Can you work these out from the model? Positions are in its coordinate system, mm. Face numbers are marked on the shaded views. A direction names the side the tool comes from. Give positions to 0.01 mm unless a question says otherwise; leave off trailing zeros. Order: outer loops, then holes, each group sorted by start corner. A loop starts at its lowest first (then second) coordinate and runs counter-clockwise, first axis right, second up. Notation, with made-up numbers: M 13.5,-23 L 55.5,-23 A24 ccw 55.5,1 Z; hole C 36.25,1 d7. An arc over 180 degrees is marked long. One line per question, with ' | ' between items. Start each with the question number.
1) Please list where these lines run through material, in increasing order: line 1 along Y through (x, z) = (0, 8.5); line 2 along X through (y, z) = (-6, 30) (3 decimals); line 3 along Y through (x, z) = (28, 38) (3 decimals). Write a range as [from, to].
2) If we section it at A-A, the plane x = 45: Please give me the cut outline in (y, z) (3 decimals).
3) Thinking about a two-plate mould opening in Y: for the marked faces 1, 2 and 3, which applies, +Y half, -Y half, draft (parallel to the pull), parting line (faces both ways), or undercut?
4) I'm going to push flat-ended pins straight in: pin 1 Ø5 at (y, z) = (5.5, 8) entering from -X; pin 2 Ø1.5 at (x, y) = (-3.5, -18) entering from +Z; pin 3 Ø15 at (y, z) = (0.5, 28.5) entering from +X (3 decimals); pin 4 Ø5 at (x, z) = (-16.5, 39.5) entering from -Y (1 decimal). Where does each tip first touch, or does it pass through?
5) If we section it at C-C, the plane z = 41: Please give me the cut outline in (x, y) (3 decimals).
6) For the marked faces 4, 5, 6, 7 and 8, which set-ups out of +Z, -Z, +X, -X, +Y, -Y let a thin tool reach every point of the face, with its end or its side?
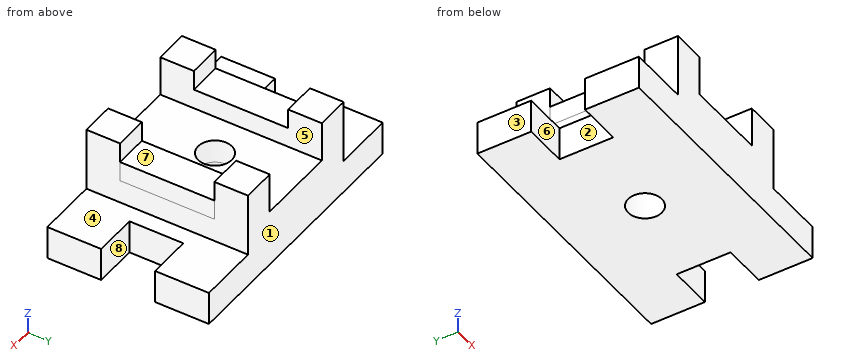
```python
from build123d import *

# Parameters (mm, degrees)
F1_DEPTH = 15.875
F2_W     = 69.85
F2_H     = 76.2
F2_R     = 7.9375
F3_DEPTH = 11.1125
F4_DEPTH = 15.876
F5_W     = 15.875
F5_H     = 15.875
F6_DEPTH = 19.05
F7_W     = 15.875
F7_H     = 44.45
F8_DEPTH = 9.525


# Not quite as in the source:
# - a length typed as a fraction of an inch, garbled in the dataset ("3 / 203.2 mm" for 3/8 in), is restored


with BuildPart() as f1:
    # F0 (on Top) → F1 (new body)
    with BuildSketch(Plane.XY):
        Polygon((63.5, 12.7), (63.5, 38.1), (-63.5, 38.1), (-63.5, 12.7), (-42.8498, 12.7), (-42.8498, -12.7), (-63.5, -12.7), (-63.5, -38.1), (63.5, -38.1), (63.5, -12.7), (42.8498, -12.7), (42.8498, 12.7), align=None)
    extrude(amount=F1_DEPTH)

    # F2 (on face) → F3 (join)
    with BuildSketch(Plane.XY.offset(15.875)):
        Rectangle(F2_W, F2_H)
        Circle(F2_R, mode=Mode.SUBTRACT)
    extrude(amount=F3_DEPTH)

    # F4 (cut, through all): a face of the model
    f4_faces = [f1.faces().sort_by_distance(p)[0] for p in [
        (0, 0, 15.875),
    ]]
    extrude(f4_faces, amount=-F4_DEPTH, mode=Mode.SUBTRACT)

    # F5 (on face) → F6 (join)
    with BuildSketch(Plane.XY.offset(26.9875)):
        with Locations((-26.9875, 30.1625)):
            Rectangle(F5_W, F5_H)
        with Locations((26.9875, 30.1625)):
            Rectangle(F5_W, F5_H)
        with Locations((26.9875, -30.1625)):
            Rectangle(F5_W, F5_H)
        with Locations((-26.9875, -30.1625)):
            Rectangle(F5_W, F5_H)
    extrude(amount=F6_DEPTH)

    # F7 (on face) → F8 (join)
    with BuildSketch(Plane.XY.offset(26.9875)):
        with Locations((26.9875, 0)):
            Rectangle(F7_W, F7_H)
        with Locations((-26.9875, 0)):
            Rectangle(F7_W, F7_H)
    extrude(amount=F8_DEPTH)


solid = f1.part
```
Results found:
1) line 1: y = [-38.1, -7.94], [7.94, 38.1] | line 2: x = [-34.925, -19.05], [19.05, 34.925] | line 3: y = [-38.1, -22.225], [22.225, 38.1]
2) outline: M -38.1,0 L -12.7,0 L -12.7,15.875 L -38.1,15.875 Z; M 12.7,0 L 38.1,0 L 38.1,15.875 L 12.7,15.875 Z
3) face 1: +Y half | face 2: undercut | face 3: draft
4) pin 1: stops at x = -42.85 | pin 2: stops at z = 26.99 | pin 3: stops at x = 34.925 | pin 4: passes through
5) outline: M -34.925,-38.1 L -19.05,-38.1 L -19.05,-22.225 L -34.925,-22.225 Z; M -34.925,22.225 L -19.05,22.225 L -19.05,38.1 L -34.925,38.1 Z; M 19.05,-38.1 L 34.925,-38.1 L 34.925,-22.225 L 19.05,-22.225 Z; M 19.05,22.225 L 34.925,22.225 L 34.925,38.1 L 19.05,38.1 Z
6) face 4: +Z, +X, +Y, -Y | face 5: +Z, +Y, -Y | face 6: +Z, -Z, -X | face 7: +Z, +X, -X | face 8: +Z, -Z, +X
